Job drawing, mm, ordinate dimensions from the low corner. One solid piece. Round coordinates to 2 decimals unless told otherwise and drop trailing zeros. Order: outer loops, then holes, each group sorted by start corner. A loop starts at its lowest first (then second) coordinate and runs counter-clockwise, first axis right, second up. Notation, with made-up numbers: (-3, 83.25) -> (29, 83.25) arc R4 ccw to (29, 87.25) -> close; hole circle Ø4 at (-39, 34.5). An arc over 180 degrees is marked (long way). Return JSON: item names as keys, results as strings. Group by question number.
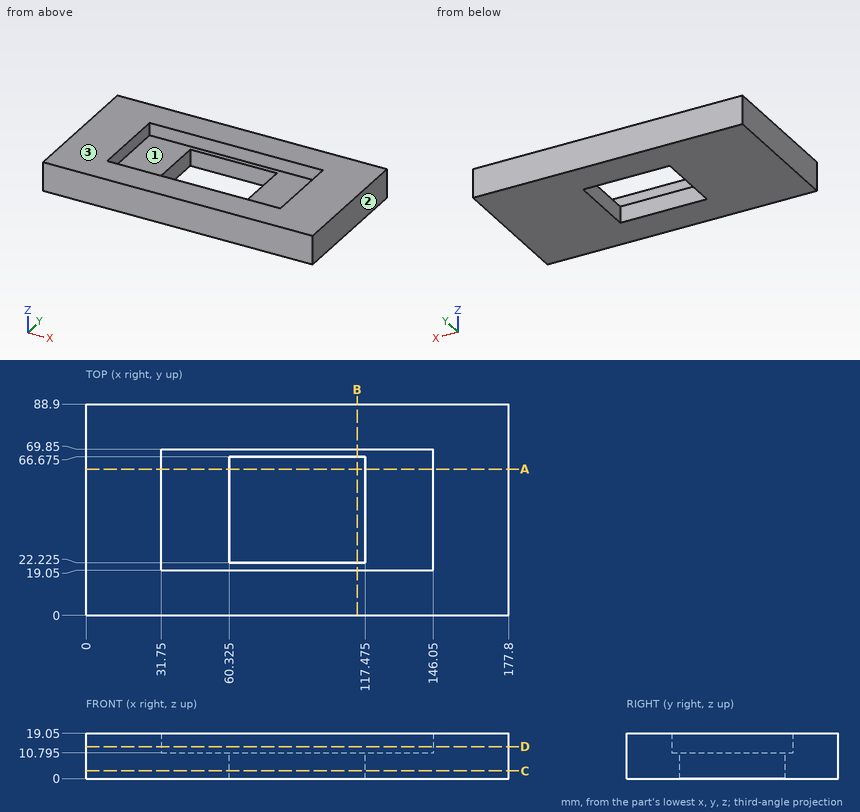
(1) Saw through at D-D, the plane z = 13.5. List the corners of the cut face in (x, y), and give its area (4 significant figures).
(2) Saw through at B-B, the plane x = 114. List the corners of the cut face in (y, z) (3 decimals), and give its area (3 significant figures).
(3) Saw through at C-C, the plane z = 3.25. List the corners of the cut face in (x, y) (3 decimals).
(4) Probe L1, parallel to Y at x = 60.5, z = 2 (3 decimals); L2, parallel to X at y = 24, z = 13.25; L3, parallel to Y at x = 133, z = 11.5. List the from-to ranges inside material, lowest first. Write a range as [from, to].
(5) Mould opens along X. For the marked faces 1, 2 and 3 say: pulls with the +X half, pulls with the -X half, needs draft (parallel to the pull), parting line crosses it, or undercut.
(6) Saw through at A-A, the plane y = 61.5. List the corners of the cut face in (x, z) (3 decimals).
Results are:
{
 "1": {"outline": "(0, 0) -> (177.8, 0) -> (177.8, 88.9) -> (0, 88.9) -> close; hole (31.75, 19.05) -> (146.05, 19.05) -> (146.05, 69.85) -> (31.75, 69.85) -> close", "area": "10,000 mm^2"},
 "2": {"outline": "(0, 0) -> (22.225, 0) -> (22.225, 10.795) -> (19.05, 10.795) -> (19.05, 19.05) -> (0, 19.05) -> close; (66.675, 0) -> (88.9, 0) -> (88.9, 19.05) -> (69.85, 19.05) -> (69.85, 10.795) -> (66.675, 10.795) -> close", "area": "794 mm^2"},
 "3": {"outline": "(0, 0) -> (177.8, 0) -> (177.8, 88.9) -> (0, 88.9) -> close; hole (60.325, 22.225) -> (117.475, 22.225) -> (117.475, 66.675) -> (60.325, 66.675) -> close"},
 "4": {"L1": "y = [0, 22.225], [66.675, 88.9]", "L2": "x = [0, 31.75], [146.05, 177.8]", "L3": "y = [0, 19.05], [69.85, 88.9]"},
 "5": {"face 1": "undercut", "face 2": "pulls with the +X half", "face 3": "needs draft"},
 "6": {"outline": "(0, 0) -> (60.325, 0) -> (60.325, 10.795) -> (31.75, 10.795) -> (31.75, 19.05) -> (0, 19.05) -> close; (117.475, 0) -> (177.8, 0) -> (177.8, 19.05) -> (146.05, 19.05) -> (146.05, 10.795) -> (117.475, 10.795) -> close"}
}
